Answer from the drawing. Dimensions are ordinates in mm from the lowest x, y and z of the part. A direction names the side the tool comes from. Give positions to 0.01 mm unless a question says otherwise; leave off trailing zeros. Loops run counter-clockwise (first coordinate to the right, second up) from the corner with the lowest first, then second, coordinate; pieces in that order, holes last.
(1) Find section C-C, the plane z = 15.25. Write down the section's boundary in (x, y), then the cut area to 3 significant figures.
(2) Find section D-D, the plane x = 11.25. Write down the section's boundary in (y, z) (1 decimal), then the cut area to 3 significant figures.
(3) Find section A-A, the plane y = 5.5. Write down the section's boundary in (x, z) (1 decimal).
(4) Straight lines are drawn through the part: probe 1 along Z at (x, y) = (25, 11) (1 decimal); probe 2 along Z at (x, y) = (2.5, 3.5) (1 decimal); probe 3 along X at (y, z) = (8.5, 23) (1 decimal). For each, find the intervals that lie inside material, in ascending order.
(5) Find section B-B, the plane y = 14.25. Write down the section's boundary in (x, z) (1 decimal), then the cut area to 3 significant figures.
(6) Each of these flat-tipped pins is pushed along its axis until it touches: P1, Ø6, axis at y = 7, z = 19.5, coming from the -X side; P2, Ø1.5, axis at x = 16, z = 17, coming from the -Y side; P3, Ø2, axis at y = 9, z = 23.5, coming from the +X side; P4, Ø2.5, axis at x = 24.9, z = 2.23, coming from the -Y side. Where does it stop, or does it pass through?
(7) Determine the mould class of the marked faces 3, 4 and 5 for opening direction X: pulls with the +X half, pulls with the -X half, needs draft (parallel to the pull), parting line crosses it, or undercut.
(8) Which of the six approach directions +Z, -Z, +X, -X, +Y, -Y give full straight-line access (tool end or side, diameter ignored) to the marked faces 1 and 2?
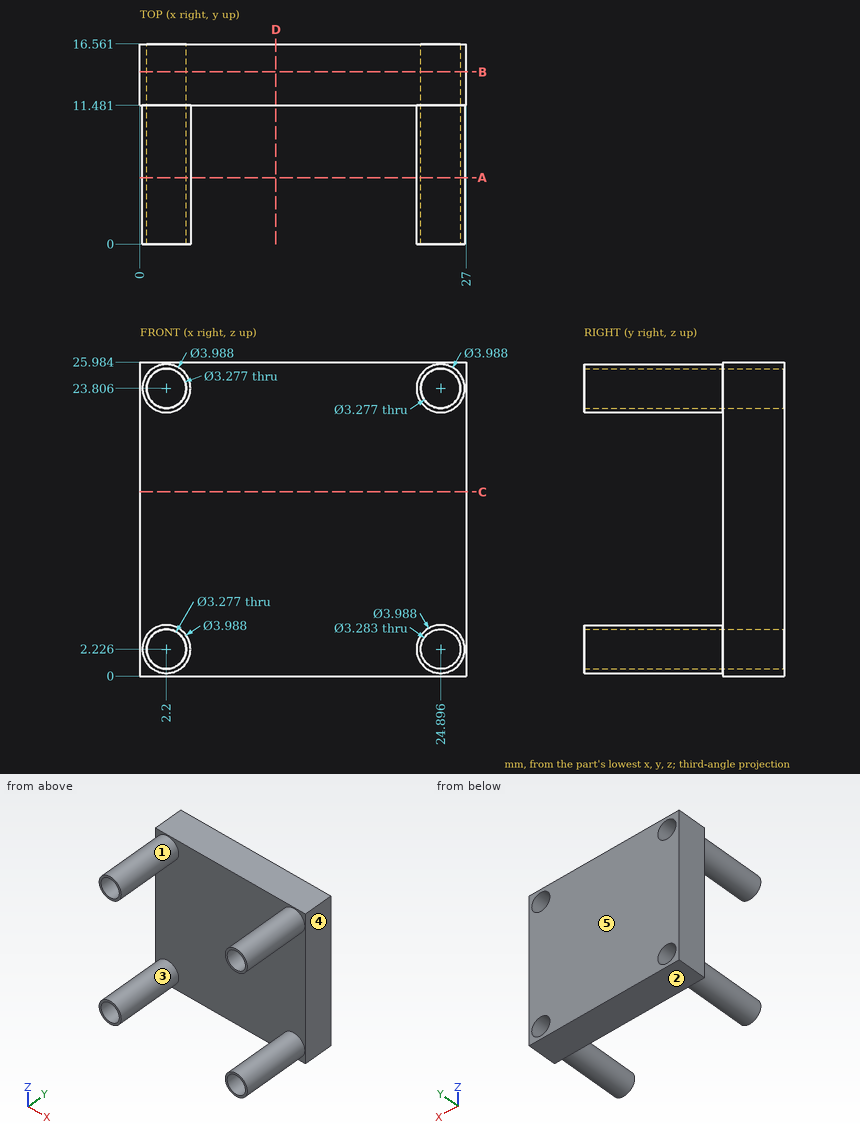
Entries:
1. outline: (0, 11.48) - (27, 11.48) - (27, 16.56) - (0, 16.56) - close
1. area: 137 mm2
2. outline: (11.5, 0) - (16.6, 0) - (16.6, 26) - (11.5, 26) - close
2. area: 132 mm2
3. outline: circle Ø4 at (2.2, 2.2); circle Ø4 at (2.2, 23.8); circle Ø4 at (24.9, 2.2); circle Ø4 at (24.9, 23.8); hole circle Ø3.3 at (2.2, 2.2); hole circle Ø3.3 at (2.2, 23.8); hole circle Ø3.3 at (24.9, 2.2); hole circle Ø3.3 at (24.9, 23.8)
4. probe 1: z = 0.2 to 0.6, 3.9 to 4.2, 21.8 to 22.2, 25.4 to 25.8
4. probe 2: z = 0.3 to 0.6, 3.8 to 4.2, 21.8 to 22.2, 25.4 to 25.8
4. probe 3: x = 0.4 to 0.8, 3.6 to 4, 23.1 to 23.5, 26.3 to 26.7
5. outline: (0, 0) - (27, 0) - (27, 26) - (0, 26) - close; hole circle Ø3.3 at (2.2, 2.2); hole circle Ø3.3 at (2.2, 23.8); hole circle Ø3.3 at (24.9, 2.2); hole circle Ø3.3 at (24.9, 23.8)
5. area: 668 mm2
6. P1: stops at x = 0.69
6. P2: stops at y = 11.48
6. P3: stops at x = 26.89
6. P4: passes through
7. face 3: undercut
7. face 4: pulls with the +X half
7. face 5: needs draft
8. face 1: -Y
8. face 2: -Z, +X, -X, +Y, -Y
